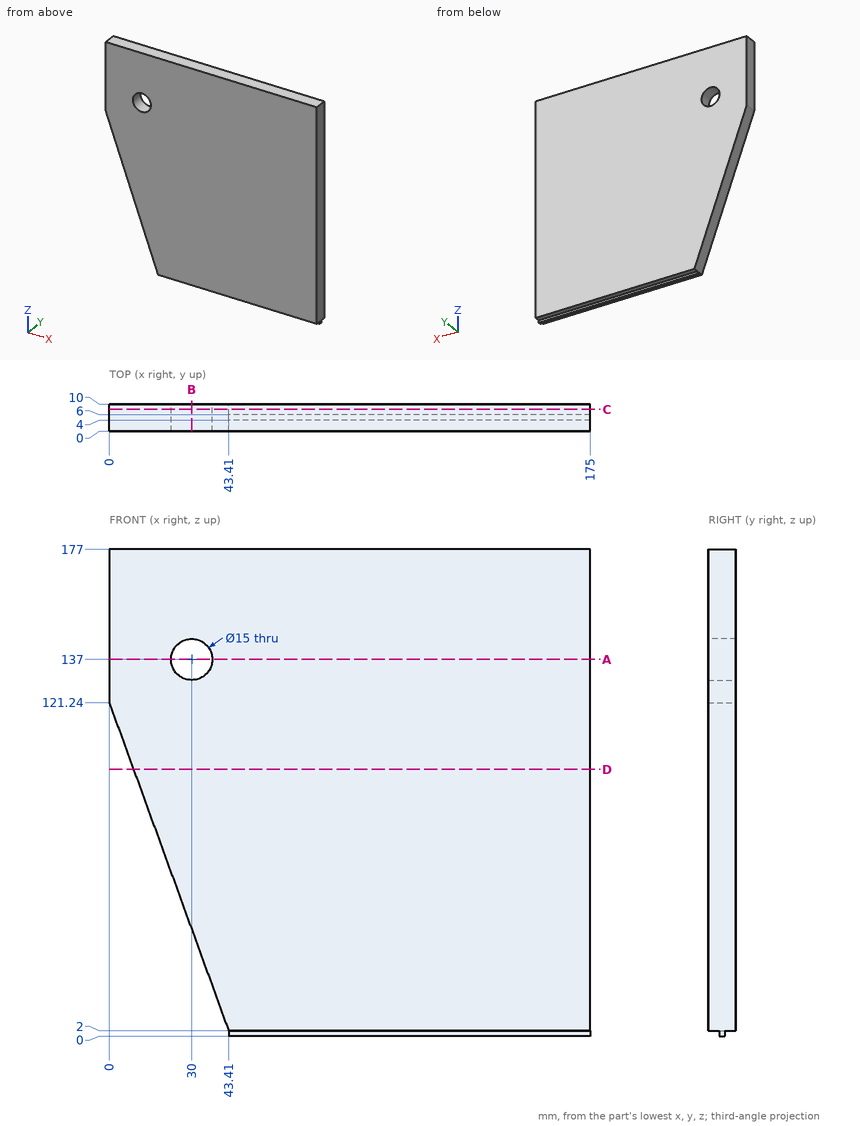
Input: dimensioned drawing with shaded views. Units: mm. Origin: part minimum x, y, z. Give positions to 0.01 mm unless a question says otherwise; leave off trailing zeros. Order: outer loops, then holes, each group sorted by start corner. A loop starts at its lowest first (then second) coordinate and runs counter-clockwise, first axis right, second up. Notation, with made-up numbers: (46, 74) -> (61, 74) arc R8 cw to (61, 84) -> close; hole circle Ø3 at (67, -12). An arc over 180 degrees is marked (long way). Use one line per item in the form item = value.
1) Section A-A, the plane z = 137. Return loops of the section in (x, y).
Response values:
outline = (0, 0) -> (22.5, 0) -> (22.5, 10) -> (0, 10) -> close; (37.5, 0) -> (175, 0) -> (175, 10) -> (37.5, 10) -> close
2) First-contact query: pin 1 Ø4.5 at (x, y) = (90, 8.5) entering from -Z; pin 2 Ø0.6 at (x, z) = (108, 0.5) entering from +Y; pin 3 Ø9 at (x, z) = (30, 137) entering from -Y; pin 4 Ø0.6 at (y, z) = (4.5, 1) entering from -X. Flat tips, straight axial feed; report the tip coordinate or a pass-through.
Response values:
pin_1 = 2
pin_2 = 6
pin_3 = through
pin_4 = 43.41
3) Section D-D, the plane z = 97. Return loops of the section in (x, y), and give its area (3 significant figures).
Response values:
outline = (8.82, 0) -> (175, 0) -> (175, 10) -> (8.82, 10) -> close
area = 1,660 mm^2
4) Section B-B, the plane x = 30. Return loops of the section in (y, z), and give its area (3 significant figures).
Response values:
outline = (0, 38.84) -> (10, 38.84) -> (10, 129.5) -> (0, 129.5) -> close; (0, 144.5) -> (10, 144.5) -> (10, 177) -> (0, 177) -> close
area = 1,230 mm^2
5) Section C-C, the plane y = 8. Return loops of the section in (x, z), and give its area (3 significant figures).
Response values:
outline = (0, 121.24) -> (43.41, 2) -> (175, 2) -> (175, 177) -> (0, 177) -> close; hole circle Ø15 at (30, 137)
area = 27,900 mm^2
6) Line query: probe 1 along X at (y, z) = (6.5, 137); probe 2 along Z at (x, y) = (55, 1.5); probe 3 along X at (y, z) = (4.75, 65.5). Output: solid intervals per line, ascending.
Response values:
probe_1 = 0 to 22.5, 37.5 to 175
probe_2 = 2 to 177
probe_3 = 20.29 to 175
